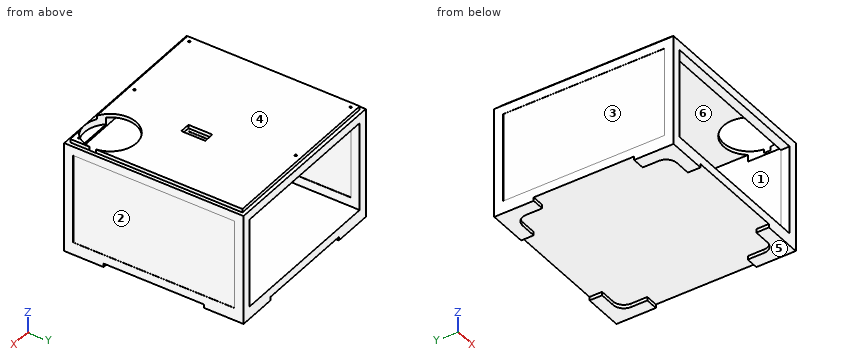
```python
from build123d import *

# Parameters (mm, degrees)
SKETCH_1_W                = 1000
SKETCH_1_H                = 1000
EXTRUDE_1_DEPTH           = 600
SKETCH_2_W                = 900
SKETCH_2_H                = 500
CUT_EXTRUDE_3_DEPTH       = 1
SKETCH_5_W                = 500
SKETCH_5_H                = 900
CUT_EXTRUDE_4_DEPTH       = 1
SKETCH_8_W                = 960
SKETCH_8_H                = 960
EXTRUDE_5_DEPTH           = 20
SKETCH_9_W                = 450
SKETCH_9_H                = 500
CUT_EXTRUDE_5_DEPTH       = 20
EXTRUDE_7_DEPTH           = 20
SKETCH_10_R               = 6
CUT_EXTRUDE_6_DEPTH       = 50
SCALE_3_SCALE             = 0.7
SKETCH_13_W               = 632
SKETCH_13_H               = 632
CUT_EXTRUDE_9_DEPTH       = 349
SKETCH_14_W               = 40.921535405
SKETCH_14_H               = 93.626348877
CUT_EXTRUDE_10_DEPTH      = 48
SKETCH_16_W               = 630
SKETCH_16_H               = 350
CUT_EXTRUDE_11_DEPTH      = 952
CUT_EXTRUDE_14_DEPTH      = 30
CUT_EXTRUDE_14_DEPTH_BACK = 41
SKETCH_17_R               = 101.559336937
SCALE_4_SCALE             = 1.3


with BuildPart() as part:
    # 草图1 → 凸台-拉伸1 (new body)
    with BuildSketch(Plane.XY):
        with Locations((450, -472.091412742)):
            Rectangle(SKETCH_1_W, SKETCH_1_H)
    extrude(amount=EXTRUDE_1_DEPTH)

    # 草图2 → 切除-拉伸3 (cut)
    with BuildSketch(Plane.XZ.offset(972.091412742)):
        with Locations((450, 300)):
            Rectangle(SKETCH_2_W, SKETCH_2_H)
    cut_extrude_3 = extrude(amount=-CUT_EXTRUDE_3_DEPTH, mode=Mode.SUBTRACT)

    # 草图5 → 切除-拉伸4 (cut)
    with BuildSketch(Plane(origin=(950, 0, 0), x_dir=(0, 0, -1), z_dir=(1, 0, 0))):
        with Locations((-300, -472.091412742)):
            Rectangle(SKETCH_5_W, SKETCH_5_H)
    cut_extrude_4 = extrude(amount=-CUT_EXTRUDE_4_DEPTH, mode=Mode.SUBTRACT)

    # 镜向1: 切除-拉伸3 across plane
    add(cut_extrude_3.mirror(Plane.ZX.offset(-472.091412742)), mode=Mode.SUBTRACT)

    # 镜向2: 切除-拉伸4 across plane
    add(cut_extrude_4.mirror(Plane.ZY.offset(-450)), mode=Mode.SUBTRACT)

    # 草图8 → 凸台-拉伸5 (add)
    with BuildSketch(Plane.XY.offset(600)):
        with Locations((450, -472.091412742)):
            Rectangle(SKETCH_8_W, SKETCH_8_H)
    extrude(amount=EXTRUDE_5_DEPTH)

    # 草图9 → 切除-拉伸5 (cut)
    with BuildSketch(Plane.XZ.offset(971.091412742)):
        with Locations((675, 300)):
            Rectangle(SKETCH_9_W, SKETCH_9_H)
    cut_extrude_5 = extrude(amount=-CUT_EXTRUDE_5_DEPTH, mode=Mode.SUBTRACT)

    # 镜向3: 切除-拉伸5 across plane
    add(cut_extrude_5.mirror(Plane.ZX.offset(-472.091412742)), mode=Mode.SUBTRACT)

    # 草图11 → 凸台-拉伸7 (add)
    with BuildSketch(Plane(origin=(0, 0, 0), x_dir=(-1, 0, 0), z_dir=(0, 0, -1))):
        with BuildLine():
            Line((-20, -192.091412742), (50, -192.091412742))
            Line((50, -192.091412742), (50, 27.908587258))
            Line((50, 27.908587258), (-170, 27.908587258))
            Line((-170, 27.908587258), (-170, -42.091412742))
            Line((-170, -42.091412742), (-80, -42.091412742))
            ThreePointArc((-80, -42.091412742), (-37.573593129, -59.665005871), (-20, -102.091412742))
            Line((-20, -102.091412742), (-20, -192.091412742))
        make_face()
        with BuildLine():
            Line((50, -972.091412742), (50, -752.091412742))
            Line((50, -752.091412742), (-20, -752.091412742))
            Line((-20, -752.091412742), (-20, -842.091412742))
            ThreePointArc((-20, -842.091412742), (-37.573593129, -884.517819614), (-80, -902.091412742))
            Line((-80, -902.091412742), (-170, -902.091412742))
            Line((-170, -902.091412742), (-170, -972.091412742))
            Line((-170, -972.091412742), (50, -972.091412742))
        make_face()
        with BuildLine():
            Line((-730, -42.091412742), (-730, 27.908587258))
            Line((-730, 27.908587258), (-950, 27.908587258))
            Line((-950, 27.908587258), (-950, -192.091412742))
            Line((-950, -192.091412742), (-880, -192.091412742))
            Line((-880, -192.091412742), (-880, -102.091412742))
            ThreePointArc((-880, -102.091412742), (-862.426406871, -59.665005871), (-820, -42.091412742))
            Line((-820, -42.091412742), (-730, -42.091412742))
        make_face()
        with BuildLine():
            Line((-950, -972.091412742), (-730, -972.091412742))
            Line((-730, -972.091412742), (-730, -902.091412742))
            Line((-730, -902.091412742), (-820, -902.091412742))
            ThreePointArc((-820, -902.091412742), (-862.426406871, -884.517819614), (-880, -842.091412742))
            Line((-880, -842.091412742), (-880, -752.091412742))
            Line((-880, -752.091412742), (-950, -752.091412742))
            Line((-950, -752.091412742), (-950, -972.091412742))
        make_face()
    extrude(amount=EXTRUDE_7_DEPTH)

    # 草图10 → 切除-拉伸6 (cut)
    with BuildSketch(Plane.XY.offset(620)):
        with Locations((450, -922.091412742)):
            Circle(SKETCH_10_R)
        with Locations((900, -922.091412742)):
            Circle(SKETCH_10_R)
        with Locations(Location((0, -922.091412742, 0), (0, 0, 180))):
            Circle(SKETCH_10_R)
        with Locations((0, -22.091412742)):
            Circle(SKETCH_10_R)
        with Locations(Location((450, -22.091412742, 0), (0, 0, 180))):
            Circle(SKETCH_10_R)
    extrude(amount=-CUT_EXTRUDE_6_DEPTH, mode=Mode.SUBTRACT)


with BuildPart() as part_1:
    # 缩放比例3: scaled about (446.683072294, -472.087239324, 308.272574941)
    add(part.part.scale(SCALE_3_SCALE).moved(Location((134.004921688, -141.626171797, 92.481772482))))

    # 草图13 → 切除-拉伸9 (cut)
    with BuildSketch(Plane.XY.offset(512.481772482)):
        with Locations((449.004921688, -472.090160717)):
            Rectangle(SKETCH_13_W, SKETCH_13_H)
    extrude(amount=-CUT_EXTRUDE_9_DEPTH, mode=Mode.SUBTRACT)

    # 草图14 → 切除-拉伸10 (cut)
    with BuildSketch(Plane.XY.offset(526.481772482)):
        with Locations((527.648380446, -489.242485135)):
            Rectangle(SKETCH_14_W, SKETCH_14_H)
    extrude(amount=-CUT_EXTRUDE_10_DEPTH, mode=Mode.SUBTRACT)

    # 草图16 → 切除-拉伸11 (cut)
    with BuildSketch(Plane(origin=(0, -122.790160717, 0), x_dir=(1, 0, 0), z_dir=(0, 1, 0))):
        with Locations((449.004921688, -302.481772482)):
            Rectangle(SKETCH_16_W, SKETCH_16_H)
    extrude(amount=-CUT_EXTRUDE_11_DEPTH, mode=Mode.SUBTRACT)

    # 草图17 → 切除-拉伸14 (cut, two sides: drawn at the far end of the back side and taken through both)
    with BuildSketch(Plane.XY.offset(526.481772482).offset(-CUT_EXTRUDE_14_DEPTH_BACK)):
        with Locations((684.208488582, -720.433496124)):
            Circle(SKETCH_17_R)
    extrude(amount=CUT_EXTRUDE_14_DEPTH + CUT_EXTRUDE_14_DEPTH_BACK, mode=Mode.SUBTRACT)


with BuildPart() as part_2:
    # 缩放比例4: scaled about (445.645805115, -468.553494774, 264.919094527)
    add(part_1.part.scale(SCALE_4_SCALE).moved(Location((-133.693741535, 140.566048432, -79.475728358))))


solid = part_2.part
```
CAD build for the part. Positions are in the model's coordinates, mm. Face numbers are marked on the shaded views. A direction names the side the tool comes from. Round coordinates to 2 decimals unless told otherwise and drop trailing zeros. Order: outer loops, then holes, each group sorted by start corner. A loop starts at its lowest first (then second) coordinate and runs counter-clockwise, first axis right, second up. Notation, with made-up numbers: (-35, 20.25) - (-8, 20.25) arc R20 ccw to (-8, 42.25) - close; hole circle Ø7 at (-33, -13). An arc over 180 degrees is marked (long way). Answer as CSV lines item,"result". Start each with the question number.
1. Pin check, flat tips, straight feed: pin 1 (9 mm diameter, centred on y = -847, z = 597.5, fed in from +X); pin 2 (4 mm diameter, centred on x = 771.5, y = -674.5, fed in from -Z); pin 3 (12 mm diameter, centred on y = -250, z = 246, fed in from -X). Stop position of each tip, or through.
2. Saw through at D-D, the plane y = -512. Write the cut outline in (x, z), and give its area (3 significant figures).
3. Pull direction Z, two halves, no side cores. Call the marked faces 4, 5 and 6: +Z half, -Z half, draft (parallel to the pull), parting line (faces both ways), or undercut.
4. Drill centre lines: L1, parallel to Z at x = 255.5, y = -361.5; L2, parallel to X at y = -481.5, z = 226; L3, parallel to Z at x = 697, y = -888.5. Where is each one in solid material? Low to high. Write a range as [from, to].
5. Saw through at C-C, the plane y = -274.5. Write the cut outline in (x, z).
6. Saw through at B-B, the plane x = 384. Write the cut outline in (y, z), and give its area (3 significant figures).
7. Saw through at A-A, the plane z = 177. Write the cut outline in (x, y).
8. Tool access for the marked faces 1, 2 and 3: list every direction of +Z, -Z, +X, -X, +Y, -Y with a clear straight run to the whole face (end or side of a thin tool).
Model answer:
1,pin 1,"stops at x = 886.81"
1,pin 2,"stops at z = 40.75"
1,pin 3,"stops at x = -4.08"
2,outline,"(-4.99, 40.75) - (905.01, 40.75) - (905.01, 86.25) - (904.1, 86.25) - (904.1, 541.25) - (905.01, 541.25) - (905.01, 586.75) - (886.81, 586.75) - (886.81, 604.95) - (578.85, 604.95) - (578.85, 586.75) - (860.81, 586.75) - (860.81, 133.05) - (859.51, 133.05) - (859.51, 86.25) - (40.51, 86.25) - (40.51, 133.05) - (39.21, 133.05) - (39.21, 586.75) - (525.65, 586.75) - (525.65, 604.95) - (13.21, 604.95) - (13.21, 586.75) - (-4.99, 586.75) - (-4.99, 541.25) - (-4.08, 541.25) - (-4.08, 86.25) - (-4.99, 86.25) - close"
2,area,"99,900 mm²"
3,face 4,"+Z half"
3,face 5,"-Z half"
3,face 6,"undercut"
4,L1,"z = [40.75, 86.25], [586.75, 604.95]"
4,L2,"x = [-4.08, 39.21], [860.81, 904.1]"
4,L3,"z = [40.75, 86.25], [541.25, 551.65]"
5,outline,"(-4.99, 40.75) - (905.01, 40.75) - (905.01, 86.25) - (904.1, 86.25) - (904.1, 541.25) - (905.01, 541.25) - (905.01, 586.75) - (886.81, 586.75) - (886.81, 604.95) - (13.21, 604.95) - (13.21, 586.75) - (-4.99, 586.75) - (-4.99, 541.25) - (-4.08, 541.25) - (-4.08, 86.25) - (-4.99, 86.25) - close; hole (39.21, 133.05) - (40.51, 133.05) - (40.51, 86.25) - (859.51, 86.25) - (859.51, 133.05) - (860.81, 133.05) - (860.81, 586.75) - (39.21, 586.75) - close"
6,outline,"(-928.15, 40.75) - (-18.15, 40.75) - (-18.15, 86.25) - (-928.15, 86.25) - close; (-928.15, 541.25) - (-883.95, 541.25) - (-883.95, 586.75) - (-62.35, 586.75) - (-62.35, 541.25) - (-18.15, 541.25) - (-18.15, 586.75) - (-36.35, 586.75) - (-36.35, 604.95) - (-909.95, 604.95) - (-909.95, 586.75) - (-928.15, 586.75) - close"
6,area,"61,300 mm²"
7,outline,"(-4.99, -928.15) - (40.51, -928.15) - (40.51, -883.95) - (39.21, -883.95) - (39.21, -62.35) - (40.51, -62.35) - (40.51, -18.15) - (-4.99, -18.15) - (-4.99, -63.65) - (-4.08, -63.65) - (-4.08, -882.65) - (-4.99, -882.65) - close; (859.51, -928.15) - (905.01, -928.15) - (905.01, -882.65) - (904.1, -882.65) - (904.1, -63.65) - (905.01, -63.65) - (905.01, -18.15) - (859.51, -18.15) - (859.51, -62.35) - (860.81, -62.35) - (860.81, -883.95) - (859.51, -883.95) - close"
8,face 1,"none"
8,face 2,"+X"
8,face 3,"-X"
